Source: three-view drawing plus pictorial views. Frame: mm from the lowest corner of the part. A direction names the side the tool comes from. Give positions to 0.01 mm unless a question says otherwise; leave off trailing zeros. Loops run counter-clockwise (first coordinate to the right, second up) from the corner with the lowest first, then second, coordinate; pieces in that order, holes last. Notation, with made-up numbers: (-30.5, 78.5) -> (23.5, 78.5) arc R25 cw to (23.5, 93.5) -> close; hole circle Ø1 at (-21, 32). An arc over 180 degrees is marked (long way). Put each result on its own line as item: value.
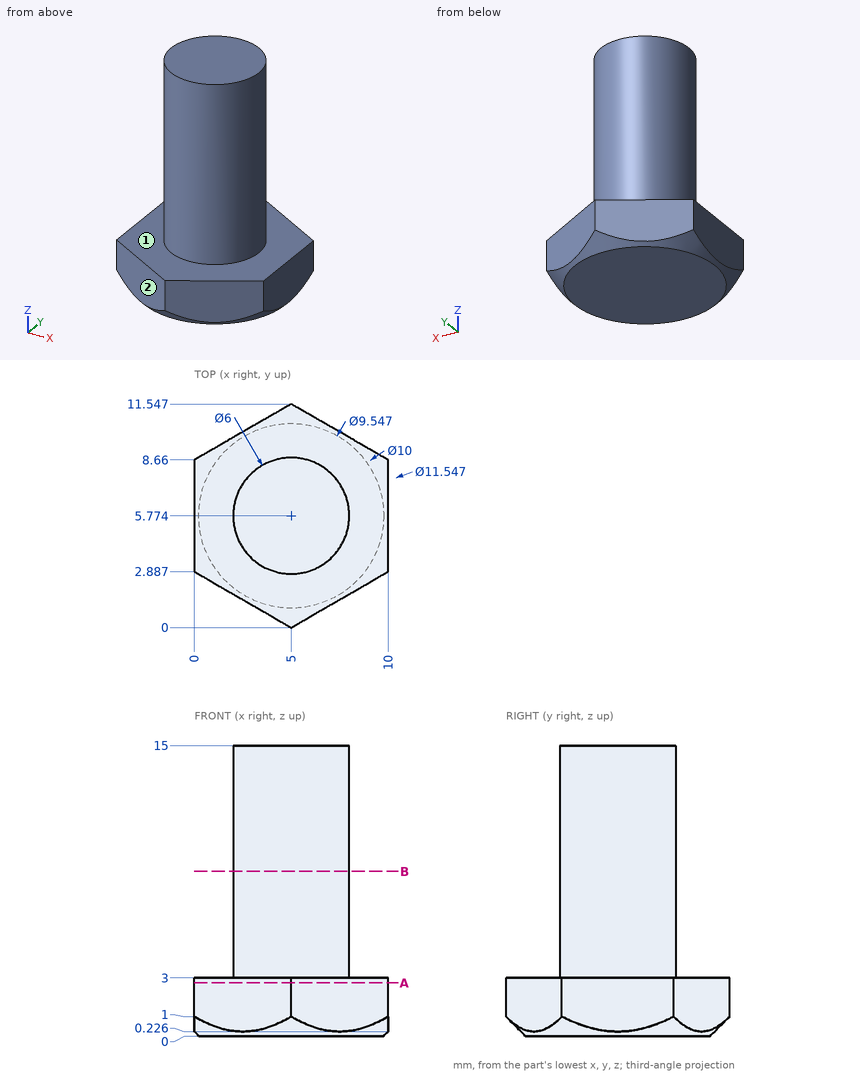
(1) Reachability of the marked faces 1 and 2 from +Z, -Z, +X, -X, +Y, -Y: full face, straight path, thin tool, end or side. Return the list, or none.
Calculated:
face 1: +Z
face 2: +Z, -Z, -X, -Y
(2) First-contact query: P1, Ø1.5, axis at x = 5, y = 1.5, coming from the +Z side; P2, Ø1.5, axis at y = 6.5, z = 7.5, coming from the -X side; P3, Ø5, axis at x = 6, z = 11.5, coming from the +Y side. Flat tips, straight axial feed; report the tip coordinate or a pass-through.
Calculated:
P1: stops at z = 3
P2: stops at x = 2
P3: stops at y = 8.77
(3) Section A-A on z = 2.75. Return loops of the section in (x, y), then the cut area to 3 significant figures.
Calculated:
outline: (0, 2.89) -> (5, 0) -> (10, 2.89) -> (10, 8.66) -> (5, 11.55) -> (0, 8.66) -> close
area: 86.6 mm²
(4) Line query: probe 1 along Y at (x, z) = (5, 6.75); probe 2 along Z at (x, y) = (6, 8.75); probe 3 along Y at (x, z) = (4.25, 13.25). Output: solid intervals per line, ascending. Write a range as from..to.
Calculated:
probe 1: y = 2.77..8.77
probe 2: z = 0..3
probe 3: y = 2.87..8.68
(5) Section B-B on z = 8.5. Return loops of the section in (x, y).
Calculated:
outline: circle Ø6 at (5, 5.77)
